Verification items for the finished model (mm, model axes). Give positions to 0.01 mm unless a question says otherwise; leave off trailing zeros. Write each loop counter-clockwise with the first axis right and the second up, starting at its lowest first coordinate (ties: lowest second). Pieces come first, ordered by that corner, then holes. Notation, with made-up numbers: (20.5, 0) - (25.5, 0) arc R24 cw to (25.5, 23) - close; hole circle Ø9 at (83, -19). An arc over 180 degrees is marked (long way). Answer as a JSON object with one key per item and string values. Group by question number.
Item 1: Sectioned sample at C-C, the plane z = 13.5. Record the boundary of the cut face in (x, y), and give its area (3 significant figures).
Item 2: Scan lines: line 1 along Y through (x, z) = (-36.35, 8.75); line 2 along Y through (x, z) = (-36.35, 26.45); line 3 along X through (y, z) = (19, 12.5). Record each from-to range of solid material in increasing order. Write a range as [from, to].
Item 3: Go/stop test with a flat-tipped pin: pin 1 (4.5 mm diameter, centred on x = 36.35, y = 27.95, fed in from +Z). Record where the tip stops, or that it passes through.
Item 4: Sectioned sample at D-D, the plane x = 36.35. Record the boundary of the cut face in (y, z), and give its area (3 significant figures).
Item 5: Sectioned sample at B-B, the plane y = -19.75. Record the boundary of the cut face in (x, z), and give its area (3 significant figures).
Item 6: Sectioned sample at A-A, the plane x = -36.35. Record the boundary of the cut face in (y, z), and give its area (3 significant figures).
```python
from build123d import *

# Parameters (mm, degrees)
F0_W      = 83
F0_H      = 65
F1_DEPTH  = 2
F2_W      = 83
F2_H      = 65
F2_R      = 2.75
F3_DEPTH  = 23
F4_R      = 2.75
F5_DEPTH  = 2.001
F6_W      = 83
F6_H      = 65
F6_R      = 2.75
F7_DEPTH  = 2
F8_W      = 10
F8_H      = 10
F9_DEPTH  = 2
F10_R     = 3
F11_DEPTH = 2


with BuildPart() as f1:
    # F0 (on Top) → F1 (new body)
    with BuildSketch(Plane.XY):
        Rectangle(F0_W, F0_H)
    extrude(amount=F1_DEPTH)

    # F2 (on face) → F3 (join)
    with BuildSketch(Plane.XY.offset(2)):
        Rectangle(F2_W, F2_H)
        with Locations((-36.35, -27.95)):
            Circle(F2_R, mode=Mode.SUBTRACT)
        with Locations((36.35, -19.75)):
            Circle(F2_R, mode=Mode.SUBTRACT)
        with Locations((-36.35, 27.95)):
            Circle(F2_R, mode=Mode.SUBTRACT)
        with BuildLine():
            Line((39.5, -30.5), (-31.196361, -30.5))
            ThreePointArc((-31.196361, -30.5), (-32.535877, -23.647098), (-39.5, -23.139595))
            Line((-39.5, -23.139595), (-39.5, 23.139595))
            ThreePointArc((-39.5, 23.139595), (-32.535877, 23.647098), (-31.196361, 30.5))
            Line((-31.196361, 30.5), (31.196361, 30.5))
            ThreePointArc((31.196361, 30.5), (32.535877, 23.647098), (39.5, 23.139595))
            Line((39.5, 23.139595), (39.5, -14.939595))
            ThreePointArc((39.5, -14.939595), (30.6, -19.75), (39.5, -24.560405))
            Line((39.5, -24.560405), (39.5, -30.5))
        make_face(mode=Mode.SUBTRACT)
        with Locations((36.35, 27.95)):
            Circle(F2_R, mode=Mode.SUBTRACT)
    extrude(amount=F3_DEPTH)

    # F4 (on face) → F5 (cut, through all)
    with BuildSketch(Plane.XY.offset(2)):
        with Locations((-36.35, 27.95)):
            Circle(F4_R)
        with Locations((-36.35, -27.95)):
            Circle(F4_R)
        with Locations((36.35, 27.95)):
            Circle(F4_R)
        with Locations((36.35, -19.75)):
            Circle(F4_R)
    extrude(amount=-F5_DEPTH, mode=Mode.SUBTRACT)

    # F6 (on face) → F7 (join)
    with BuildSketch(Plane.XY.offset(25)):
        Rectangle(F6_W, F6_H)
        with Locations((-36.35, -27.95)):
            Circle(F6_R, mode=Mode.SUBTRACT)
        with Locations((36.35, -19.75)):
            Circle(F6_R, mode=Mode.SUBTRACT)
        with Locations((-36.35, 27.95)):
            Circle(F6_R, mode=Mode.SUBTRACT)
        with Locations((36.35, 27.95)):
            Circle(F6_R, mode=Mode.SUBTRACT)
    extrude(amount=F7_DEPTH)

    # F8 (on face) → F9 (cut)
    with BuildSketch(Plane.YZ.offset(41.5)):
        with Locations((4.1, 13.5)):
            Rectangle(F8_W, F8_H)
    extrude(amount=-F9_DEPTH, mode=Mode.SUBTRACT)

    # F10 (on face) → F11 (cut)
    with BuildSketch(Plane(origin=(-41.5, 0, 0), x_dir=(0, -1, 0), z_dir=(-1, 0, 0))):
        with Locations((0, 13.5)):
            Circle(F10_R)
    extrude(amount=-F11_DEPTH, mode=Mode.SUBTRACT)


solid = f1.part
```
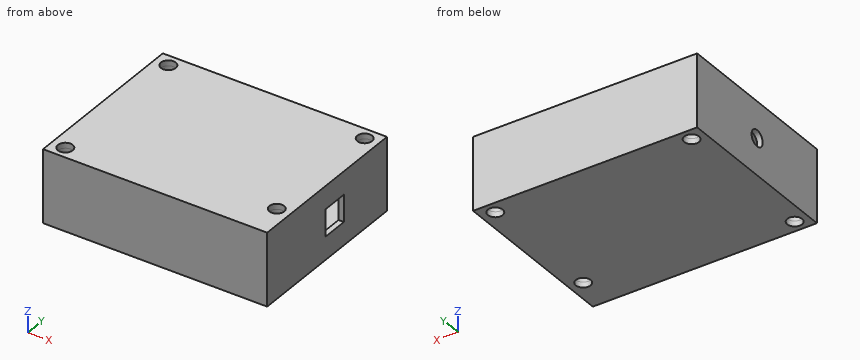
Geometry check:
{
 "1": {"outline": "(-41.5, -32.5) - (41.5, -32.5) - (41.5, -0.9) - (39.5, -0.9) - (39.5, -14.94) arc R5.75 ccw (long way) to (39.5, -24.56) - (39.5, -30.5) - (-31.2, -30.5) arc R5.75 ccw to (-39.5, -23.14) - (-39.5, -3) - (-41.5, -3) - close; (-41.5, 3) - (-39.5, 3) - (-39.5, 23.14) arc R5.75 ccw to (-31.2, 30.5) - (31.2, 30.5) arc R5.75 ccw to (39.5, 23.14) - (39.5, 9.1) - (41.5, 9.1) - (41.5, 32.5) - (-41.5, 32.5) - close; hole circle Ø5.5 at (-36.35, -27.95); hole circle Ø5.5 at (-36.35, 27.95); hole circle Ø5.5 at (36.35, -19.75); hole circle Ø5.5 at (36.35, 27.95)", "area": "731 mm^2"},
 "2": {"line 1": "[-32.5, -30.7], [-25.2, -22.2], [22.2, 25.2], [30.7, 32.5]", "line 2": "[-32.5, -30.7], [-25.2, 25.2], [30.7, 32.5]", "line 3": "[-41.5, -39.5], [39.5, 41.5]"},
 "3": {"pin 1": "through"},
 "4": {"outline": "(-32.5, 0) - (-22.5, 0) - (-22.5, 27) - (-32.5, 27) - close; (-17, 0) - (25.2, 0) - (25.2, 27) - (-17, 27) - close; (30.7, 0) - (32.5, 0) - (32.5, 27) - (30.7, 27) - close; hole (-30.5, 2) - (-25.5, 2) - (-25.5, 25) - (-30.5, 25) - close; hole (-14, 2) - (22.2, 2) - (22.2, 25) - (-14, 25) - close", "area": "510 mm^2"},
 "5": {"outline": "(-41.5, 0) - (33.6, 0) - (33.6, 27) - (-41.5, 27) - close; (39.1, 0) - (41.5, 0) - (41.5, 27) - (39.1, 27) - close; hole (-39.5, 2) - (30.6, 2) - (30.6, 25) - (-39.5, 25) - close", "area": "480 mm^2"},
 "6": {"outline": "(-32.5, 0) - (-30.7, 0) - (-30.7, 27) - (-32.5, 27) - close; (-25.2, 0) - (25.2, 0) - (25.2, 27) - (-25.2, 27) - close; (30.7, 0) - (32.5, 0) - (32.5, 27) - (30.7, 27) - close; hole (-22.2, 2) - (22.2, 2) - (22.2, 25) - (-22.2, 25) - close", "area": "437 mm^2"}
}
